from build123d import *

# Parameters (mm, degrees)
F0_R     = 1.7
F1_DEPTH = 5
F2_DEPTH = 8
F3_DEPTH = 17
F4_R     = 2.3
F5_DEPTH = 25


with BuildPart() as f1:
    # F0 (on Front) → F1 (new body)
    with BuildSketch(Plane.XZ):
        with BuildLine():
            ThreePointArc((4.1207105035, 10.4681538462), (9.2984002163, 6.3326340032), (11.25, 0))
            ThreePointArc((11.25, 0), (8.6331483249, -7.2132690231), (2, -11.0707949127))
            Line((2, -11.0707949127), (2, -18.75))
            Line((2, -18.75), (10, -18.75))
            ThreePointArc((10, -18.75), (16.0767582704, -13.8960549623), (20, -7.1807033082))
            ThreePointArc((20, -7.1807033082), (20.9351677806, -3.6443449343), (21.25, 0))
            ThreePointArc((21.25, 0), (16.9251932479, 12.8491374621), (5.7111450805, 20.4681538462))
            ThreePointArc((5.7111450805, 20.4681538462), (6.7438538712, 18.470458278), (7.1, 16.25))
            ThreePointArc((7.1, 16.25), (6.3113803789, 12.9978502936), (4.1207105035, 10.4681538462))
        make_face()
        with BuildLine():
            ThreePointArc((2, 11.0707949127), (3.0751533833, 10.8215494117), (4.1207105035, 10.4681538462))
            ThreePointArc((4.1207105035, 10.4681538462), (6.3113803789, 12.9978502936), (7.1, 16.25))
            ThreePointArc((7.1, 16.25), (6.7438538712, 18.470458278), (5.7111450805, 20.4681538462))
            ThreePointArc((5.7111450805, 20.4681538462), (3.4504663185, 20.9679942337), (1.1488269912, 21.2189230769))
            ThreePointArc((1.1488269912, 21.2189230769), (3.9918052091, 19.4241914203), (5.1, 16.25))
            ThreePointArc((5.1, 16.25), (3.8904803589, 12.9524004827), (0.8356225189, 11.2189230769))
            ThreePointArc((0.8356225189, 11.2189230769), (1.4197444332, 11.1600549167), (2, 11.0707949127))
        make_face()
        with BuildLine():
            ThreePointArc((-0.8356225189, 11.2189230769), (0, 11.25), (0.8356225189, 11.2189230769))
            ThreePointArc((0.8356225189, 11.2189230769), (3.8904803589, 12.9524004827), (5.1, 16.25))
            ThreePointArc((5.1, 16.25), (3.9918052091, 19.4241914203), (1.1488269912, 21.2189230769))
            ThreePointArc((1.1488269912, 21.2189230769), (0, 21.25), (-1.1488269912, 21.2189230769))
            ThreePointArc((-1.1488269912, 21.2189230769), (-5.0975003643, 16.0903440089), (-0.8356225189, 11.2189230769))
        make_face()
        with Locations((0, 16.25)):
            Circle(F0_R, mode=Mode.SUBTRACT)
        with BuildLine():
            ThreePointArc((2, -11.0707949127), (8.6331483249, -7.2132690231), (11.25, 0))
            ThreePointArc((11.25, 0), (9.2984002163, 6.3326340032), (4.1207105035, 10.4681538462))
            ThreePointArc((4.1207105035, 10.4681538462), (3.1034384471, 9.864182135), (2, 9.4375114679))
            Line((2, 9.4375114679), (2, 8.7749643874))
            ThreePointArc((2, 8.7749643874), (7.0356236397, 5.6124860802), (9, 0))
            ThreePointArc((9, 0), (7.0356236397, -5.6124860802), (2, -8.7749643874))
            Line((2, -8.7749643874), (2, -11.0707949127))
        make_face()
        with BuildLine():
            ThreePointArc((2, 9.4375114679), (3.1034384471, 9.864182135), (4.1207105035, 10.4681538462))
            ThreePointArc((4.1207105035, 10.4681538462), (3.0751533833, 10.8215494117), (2, 11.0707949127))
            Line((2, 11.0707949127), (2, 9.4375114679))
        make_face()
        with BuildLine():
            ThreePointArc((20, -7.1807033082), (16.0767582704, -13.8960549623), (10, -18.75))
            Line((10, -18.75), (10, -66.05))
            Line((10, -66.05), (20, -66.05))
            Line((20, -66.05), (20, -7.1807033082))
        make_face()
    extrude(amount=F1_DEPTH)

    # F0 (on Front) → F2 (join)
    with BuildSketch(Plane.XZ):
        with BuildLine():
            ThreePointArc((4.1207105035, 10.4681538462), (9.2984002163, 6.3326340032), (11.25, 0))
            ThreePointArc((11.25, 0), (8.6331483249, -7.2132690231), (2, -11.0707949127))
            Line((2, -11.0707949127), (2, -18.75))
            Line((2, -18.75), (10, -18.75))
            ThreePointArc((10, -18.75), (16.0767582704, -13.8960549623), (20, -7.1807033082))
            ThreePointArc((20, -7.1807033082), (20.9351677806, -3.6443449343), (21.25, 0))
            ThreePointArc((21.25, 0), (16.9251932479, 12.8491374621), (5.7111450805, 20.4681538462))
            ThreePointArc((5.7111450805, 20.4681538462), (6.7438538712, 18.470458278), (7.1, 16.25))
            ThreePointArc((7.1, 16.25), (6.3113803789, 12.9978502936), (4.1207105035, 10.4681538462))
        make_face()
        with BuildLine():
            ThreePointArc((2, 11.0707949127), (3.0751533833, 10.8215494117), (4.1207105035, 10.4681538462))
            ThreePointArc((4.1207105035, 10.4681538462), (6.3113803789, 12.9978502936), (7.1, 16.25))
            ThreePointArc((7.1, 16.25), (6.7438538712, 18.470458278), (5.7111450805, 20.4681538462))
            ThreePointArc((5.7111450805, 20.4681538462), (3.4504663185, 20.9679942337), (1.1488269912, 21.2189230769))
            ThreePointArc((1.1488269912, 21.2189230769), (3.9918052091, 19.4241914203), (5.1, 16.25))
            ThreePointArc((5.1, 16.25), (3.8904803589, 12.9524004827), (0.8356225189, 11.2189230769))
            ThreePointArc((0.8356225189, 11.2189230769), (1.4197444332, 11.1600549167), (2, 11.0707949127))
        make_face()
        with BuildLine():
            ThreePointArc((-0.8356225189, 11.2189230769), (0, 11.25), (0.8356225189, 11.2189230769))
            ThreePointArc((0.8356225189, 11.2189230769), (3.8904803589, 12.9524004827), (5.1, 16.25))
            ThreePointArc((5.1, 16.25), (3.9918052091, 19.4241914203), (1.1488269912, 21.2189230769))
            ThreePointArc((1.1488269912, 21.2189230769), (0, 21.25), (-1.1488269912, 21.2189230769))
            ThreePointArc((-1.1488269912, 21.2189230769), (-5.0975003643, 16.0903440089), (-0.8356225189, 11.2189230769))
        make_face()
        with Locations((0, 16.25)):
            Circle(F0_R, mode=Mode.SUBTRACT)
        with BuildLine():
            ThreePointArc((20, -7.1807033082), (16.0767582704, -13.8960549623), (10, -18.75))
            Line((10, -18.75), (10, -66.05))
            Line((10, -66.05), (20, -66.05))
            Line((20, -66.05), (20, -7.1807033082))
        make_face()
    extrude(amount=F2_DEPTH)

    # F0 (on Front) → F3 (join)
    with BuildSketch(Plane.XZ):
        with BuildLine():
            ThreePointArc((20, -7.1807033082), (16.0767582704, -13.8960549623), (10, -18.75))
            Line((10, -18.75), (10, -66.05))
            Line((10, -66.05), (20, -66.05))
            Line((20, -66.05), (20, -7.1807033082))
        make_face()
        with BuildLine():
            ThreePointArc((4.1207105035, 10.4681538462), (9.2984002163, 6.3326340032), (11.25, 0))
            ThreePointArc((11.25, 0), (8.6331483249, -7.2132690231), (2, -11.0707949127))
            Line((2, -11.0707949127), (2, -18.75))
            Line((2, -18.75), (10, -18.75))
            ThreePointArc((10, -18.75), (16.0767582704, -13.8960549623), (20, -7.1807033082))
            ThreePointArc((20, -7.1807033082), (20.9351677806, -3.6443449343), (21.25, 0))
            ThreePointArc((21.25, 0), (16.9251932479, 12.8491374621), (5.7111450805, 20.4681538462))
            ThreePointArc((5.7111450805, 20.4681538462), (6.7438538712, 18.470458278), (7.1, 16.25))
            ThreePointArc((7.1, 16.25), (6.3113803789, 12.9978502936), (4.1207105035, 10.4681538462))
        make_face()
    extrude(amount=F3_DEPTH)

    # F4 (on face) → F5 (cut)
    with BuildSketch(Plane.YZ.offset(20)):
        with Locations((-8.5, -56.05)):
            Circle(F4_R)
        with Locations((-8.5, -36.05)):
            Circle(F4_R)
    extrude(amount=-F5_DEPTH, mode=Mode.SUBTRACT)


solid = f1.part
Can you work these out from the model? Positions are in its coordinate system, mm. A direction names the side the tool comes from. Give positions to 0.01 mm unless a question says otherwise; leave off trailing zeros. Write each loop counter-clockwise with the first axis right and the second up, starting at its lowest first coordinate (ties: lowest second). Pieces come first, ordered by that corner, then holes. Notation, with made-up numbers: M 10.25,77.25 L 21.25,77.25 A25 cw 21.25,99.25 Z; hole C -17,-20.5 d11. An arc over 180 degrees is marked long. Answer in a Markdown table with one row per item. Add a question column.
Item 1: Imagine slicing it at C-C, the plane y = -16. Write out the boundary of the cut face in (x, z).
Item 2: Please list where these lines run through material, in increasing order: L1, parallel to Z at x = 16.75, y = -8.5; L2, parallel to Z at x = 14, y = -7.5; L3, parallel to Z at x = 0, y = -3.5.
Item 3: We'd pull the mould along Z, two halves only. Please class faces 1 (the flat face through (2, -2, 10)), 2 (the flat face through (15, -8, -66.05)), 3 (the flat face through (9.3, -5, 0.1)): released by +Z, released by -Z, zero draft, split by the parting line, or undercut.
Item 4: On a 3-axis mill with a long thin cutter (end or side, diameter ignored), from which of +Z, -Z, +X, -X, +Y, -Y can I reach the whole of each face in a straight line? I mean faces 4 (the flat face through (2, -8, -15)), 5 (the flat face through (14, -17, -22)), 6 (the flat face through (20, -5, -37)). Say none if no direction works.
Item 5: Imagine slicing it at D-D, the plane y = -1.75. Write out the boundary of the cut face in (x, z).
Item 6: Imagine slicing it at B-B, the plane x = 0. Write out the boundary of the cut face in (y, z), plus the area to 3 significant figures.
Item 7: Imagine slicing it at A-A, the plane z = -36.05. Write out the boundary of the cut face in (x, y), plus the area to 3 significant figures.
Item 8: For pin 1 Ø1 at (y, z) = (-13, -3.5) entering from -X; pin 2 Ø4 at (x, y) = (6, -8) entering from +Z; pin 3 Ø2 at (y, z) = (-14, 7) entering from -X, each with a flat end and sliding along its axis, tell me the tip position at first contact or that it passes through.
Evaluation:
| question | item | result |
|---|---|---|
| 1 | outline | M 2,-18.75 L 10,-18.75 L 10,-66.05 L 20,-66.05 L 20,-7.18 A21.25 ccw 5.71,20.47 A7.1 cw 4.12,10.47 A11.25 cw 2,-11.07 Z |
| 2 | L1 | z = -66.05 to -58.35, -53.75 to -38.35, -33.75 to 13.08 |
| 2 | L2 | z = -66.05 to -58.12, -53.98 to -38.12, -33.98 to 15.99 |
| 2 | L3 | z = 11.25 to 14.55, 17.95 to 21.25 |
| 3 | face 1 | zero draft |
| 3 | face 2 | released by -Z |
| 3 | face 3 | undercut |
| 4 | face 4 | -Z, -X, +Y, -Y |
| 4 | face 5 | +Z, -Z, +X, -X, -Y |
| 4 | face 6 | -Z, +X, +Y, -Y |
| 5 | outline | M -1.15,21.22 A5.1 ccw -0.84,11.22 A11.25 cw 2,11.07 L 2,8.77 A9 cw 2,-8.77 L 2,-18.75 L 10,-18.75 L 10,-66.05 L 20,-66.05 L 20,-7.18 A21.25 ccw Z; hole C 0,16.25 d3.4 |
| 6 | outline | M -8,11.25 L 0,11.25 L 0,14.55 L -8,14.55 Z; M -8,17.95 L 0,17.95 L 0,21.25 L -8,21.25 Z |
| 6 | area | 52.8 mm² |
| 7 | outline | M 10,-17 L 20,-17 L 20,-10.8 L 10,-10.8 Z; M 10,-6.2 L 20,-6.2 L 20,0 L 10,0 Z |
| 7 | area | 124 mm² |
| 8 | pin 1 | stops at x = 10.51 |
| 8 | pin 2 | stops at z = 20.87 |
| 8 | pin 3 | stops at x = 7.91 |
